```python
from build123d import *

# Parameters (mm, degrees)
F0_R          = 1.5
F1_DEPTH      = 35
F3_DEPTH      = 20.992492
F3_DEPTH_BACK = 20.992492


with BuildPart() as f1:
    # F0 (on Top) → F1 (new body)
    with BuildSketch(Plane.XY):
        with BuildLine():
            Line((12.991492, 14.542047), (11.5, 0))
            ThreePointArc((11.5, 0), (0, -11.5), (-11.5, 0))
            Line((-11.5, 0), (-12.991492, 14.542047))
            Line((-12.991492, 14.542047), (-13.074771, 15.354019))
            ThreePointArc((-13.074771, 15.354019), (-17.399607, 18.521173), (-20.991492, 14.542047))
            Line((-20.991492, 14.542047), (-19.094014, -3.95836))
            ThreePointArc((-19.094014, -3.95836), (-12.309792, -15.123459), (0, -19.5))
            ThreePointArc((0, -19.5), (12.309792, -15.123459), (19.094014, -3.95836))
            Line((19.094014, -3.95836), (20.991492, 14.542047))
            ThreePointArc((20.991492, 14.542047), (17.399607, 18.521173), (13.074771, 15.354019))
            Line((13.074771, 15.354019), (12.991492, 14.542047))
        make_face()
        with Locations((0, -15.5)):
            Circle(F0_R, mode=Mode.SUBTRACT)
        with Locations((-16.686909, 11.367775)):
            Circle(F0_R, mode=Mode.SUBTRACT)
        with Locations((16.686909, 11.367775)):
            Circle(F0_R, mode=Mode.SUBTRACT)
    extrude(amount=F1_DEPTH)

    # F2 (on Right) → F3 (cut, two sides)
    with BuildSketch(Plane.YZ) as f3_sk:
        Polygon((18.542047, 35), (14.542047, 35), (-3.95836, 35), (18.542047, 20), align=None)
    extrude(amount=F3_DEPTH, mode=Mode.SUBTRACT)
    extrude(f3_sk.sketch, amount=-F3_DEPTH_BACK, mode=Mode.SUBTRACT)


solid = f1.part
```
The listing builds one solid part. Answer for the finished solid, in the listing's coordinates (mm). Give positions to 0.01 mm unless a question says otherwise; leave off trailing zeros. Order: outer loops, then holes, each group sorted by start corner. A loop starts at its lowest first (then second) coordinate and runs counter-clockwise, first axis right, second up.
1) Find section D-D on z = 16. Write down the section's boundary in (x, y), then the cut area to 3 significant figures.
Reported:
outline: (-20.99, 14.54) - (-19.09, -3.96) arc R19.5 ccw to (19.09, -3.96) - (20.99, 14.54) arc R4 ccw to (13.07, 15.35) - (12.99, 14.54) - (11.5, 0) arc R11.5 cw to (-11.5, 0) - (-12.99, 14.54) - (-13.07, 15.35) arc R4 ccw to start; hole circle Ø3 at (-16.69, 11.37); hole circle Ø3 at (0, -15.5); hole circle Ø3 at (16.69, 11.37)
area: 651 mm2
2) Given P1, Ø2, axis at x = -3, z = 14.5, coming from the +Y side; P2, Ø5, axis at x = -10, z = 27.5, coming from the -Y side; P3, Ø5, axis at x = 6, z = 24, coming from the -Y side; P4, Ø1.8, axis at x = 16.69, y = 11.37, coming from the -Z side, each flat-ended and moving along its own axis, determine where each tip first touches the part or whether it passes through.
Reported:
P1: stops at y = -10.78
P2: stops at y = -18
P3: stops at y = -19.18
P4: passes through
3) Find section C-C on y = -15.5. Write down the section's boundary in (x, z), then the cut area to 3 significant figures.
Reported:
outline: (-11.83, 0) - (-1.5, 0) - (-1.5, 35) - (-11.83, 35) - close; (1.5, 0) - (11.83, 0) - (11.83, 35) - (1.5, 35) - close
area: 723 mm2
4) Find section A-A on x = -16. Write down the section's boundary in (y, z).
Reported:
outline: (-11.15, 0) - (10.03, 0) - (10.03, 25.67) - (-3.96, 35) - (-11.15, 35) - close; (12.7, 0) - (18.42, 0) - (18.42, 20.08) - (12.7, 23.89) - close
5) Find section B-B on z = 30. Write down the section's boundary in (x, y), then the cut area to 3 significant figures.
Reported:
outline: (-19.86, 3.54) - (-19.09, -3.96) arc R19.5 ccw to (19.09, -3.96) - (19.86, 3.54) - (11.86, 3.54) - (11.5, 0) arc R11.5 cw to (-11.5, 0) - (-11.86, 3.54) - close; hole circle Ø3 at (0, -15.5)
area: 439 mm2
6) Consider line 1 along X through (y, z) = (11.5, 22.5); line 2 along X through (y, z) = (14.5, 9.5); line 3 along X through (y, z) = (7, 19.5). Determine where each line is inside the solid, lowest interval first.
Reported:
line 1: x = -20.68 to -18.18, -15.19 to -12.68, 12.68 to 15.19, 18.18 to 20.68
line 2: x = -20.99 to -12.99, 12.99 to 20.99
line 3: x = -20.22 to -12.22, 12.22 to 20.22
7) Determine the mould class of faces 1 (the face through (0, -12, 35)), 2 (the face through (-20.056, 5.421, 13.366)), 3 (the face through (16.362, 9.903, 12.723)), 4 (the face through (-17, 9.9, 12.7)) for opening direction Y: pulls with the +Y half, pulls with the -Y half, needs draft (parallel to the pull), parting line crosses it, or undercut.
Reported:
face 1: needs draft
face 2: pulls with the -Y half
face 3: undercut
face 4: undercut
